Geometry check sheet. Reference: drawing and pictorial views, mm from the part's lowest x, y, z. A direction names the side the tool comes from. Give positions to 0.01 mm unless a question says otherwise; leave off trailing zeros. Write each loop counter-clockwise with the first axis right and the second up, starting at its lowest first coordinate (ties: lowest second). Pieces come first, ordered by that corner, then holes. Notation, with made-up numbers: M 44,-19.75 L 98,-19.75 A20 cw 98,-7.75 Z; hole C 81.5,7.25 d5. An arc over 180 degrees is marked long. One line per item, written item: value. Start each with the question number.
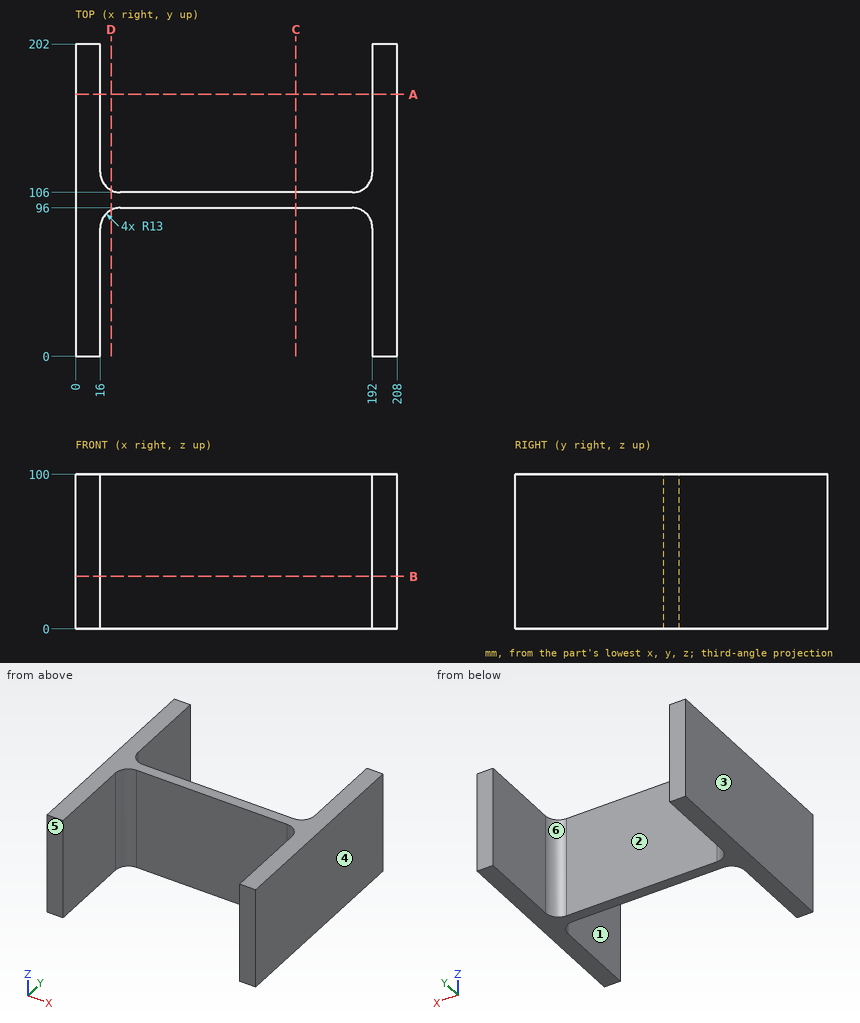
1) Cross-section at D-D (x = 23). Record the boundary of the cut face in (y, z), plus the area to 3 significant figures.
2) Cross-section at C-C (x = 142.5). Record the boundary of the cut face in (y, z).
3) Cross-section at A-A (y = 169.5). Record the boundary of the cut face in (x, z).
4) Material ranges on L1, parallel to X at y = 39.5, z = 56; L2, parallel to Y at x = 148, z = 37; L3, parallel to Y at x = 27.5, z = 13, recorded low to high. Write a range as from..to.
5) Cross-section at B-B (z = 34). Record the boundary of the cut face in (x, y).
6) Draft check along X on the marked faces 4, 5 and 6. Enter one of: released by +X, released by -X, zero draft, split by the parting line, or undercut.
7) Gauge pin test, flat ends, axial feed: pin 1 (5 mm diameter, centred on x = 119.5, z = 74.5, fed in from +Y); pin 2 (8 mm diameter, centred on x = 51.5, z = 38.5, fed in from -Y); pin 3 (12 mm diameter, centred on x = 31.5, z = 52, fed in from -Y). Record the tip position at first contact, or that the pin passes through.
8) Tool access check on the marked faces 1, 2 and 3. Record the directions out of +Z, -Z, +X, -X, +Y, -Y that give a thin tool (end or side, any length) a straight path to the whole face; none if there is none.
Data:
1. outline: M 94.53,0 L 107.47,0 L 107.47,100 L 94.53,100 Z
1. area: 1,290 mm2
2. outline: M 96,0 L 106,0 L 106,100 L 96,100 Z
3. outline: M 0,0 L 16,0 L 16,100 L 0,100 Z; M 192,0 L 208,0 L 208,100 L 192,100 Z
4. L1: x = 0..16, 192..208
4. L2: y = 96..106
4. L3: y = 95.91..106.09
5. outline: M 0,0 L 16,0 L 16,83 A13 cw 29,96 L 179,96 A13 cw 192,83 L 192,0 L 208,0 L 208,202 L 192,202 L 192,119 A13 cw 179,106 L 29,106 A13 cw 16,119 L 16,202 L 0,202 Z
6. face 4: released by +X
6. face 5: zero draft
6. face 6: undercut
7. pin 1: stops at y = 106
7. pin 2: stops at y = 96
7. pin 3: stops at y = 95.52
8. face 1: +Z, -Z, -Y
8. face 2: +Z, -Z, +Y
8. face 3: +Z, -Z, -X, +Y, -Y
